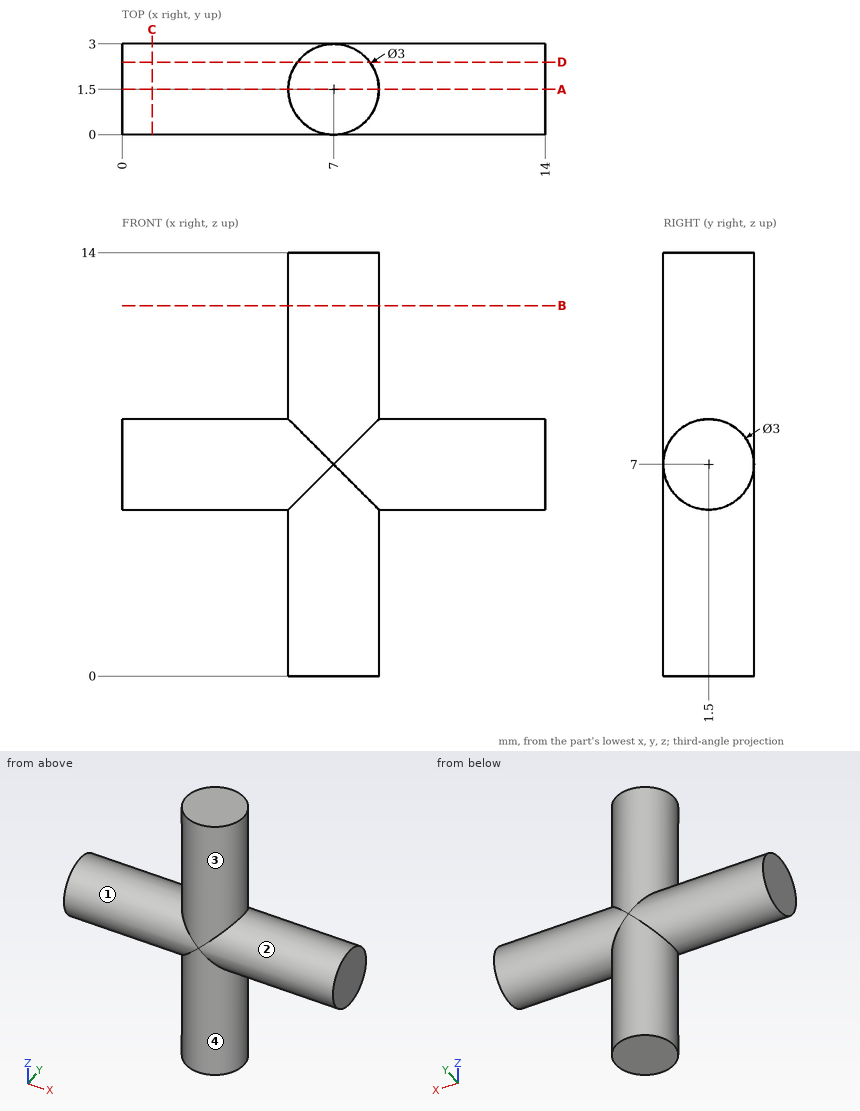
Check sheet for the drawn part. Datum: minimum x, y, z corner. Units: mm. A direction names the side the tool comes from. Coordinates: 2 decimals unless noted, no trailing zeros. Loops run counter-clockwise (first coordinate to the right, second up) from the corner with the lowest first, then second, coordinate; pieces in that order, holes last. Notation, with made-up numbers: (5, -8.5) - (62, -8.5) arc R14 ccw to (62, 9.5) - close; hole circle Ø3 at (-30, 55). An arc over 180 degrees is marked (long way). Put each result on its own line as item: value.
Item 1: Gauge pin test, flat end, axial feed: pin 1 Ø1 at (x, z) = (4, 1.5) entering from +Y. Record the tip position at first contact, or that the pin passes through.
Conclusion:
pin 1: passes through
Item 2: Set-up check for the marked faces 1, 2, 3 and 4: record each of +Z, -Z, +X, -X, +Y, -Y from which the full face is reachable in a straight line by a thin tool's end or side.
Conclusion:
face 1: -X
face 2: +X
face 3: +Z
face 4: -Z
Item 3: Section check C-C (x = 1). Enter the section's corners in (y, z), then the cut area to 3 significant figures.
Conclusion:
outline: circle Ø3 at (1.5, 7)
area: 7.07 mm2
Item 4: Section check A-A (y = 1.5). Enter the section's corners in (x, z).
Conclusion:
outline: (0, 5.5) - (5.5, 5.5) - (5.5, 0) - (8.5, 0) - (8.5, 5.5) - (14, 5.5) - (14, 8.5) - (8.5, 8.5) - (8.5, 14) - (5.5, 14) - (5.5, 8.5) - (0, 8.5) - close
Item 5: Section check D-D (y = 2.4). Enter the section's corners in (x, z).
Conclusion:
outline: (0, 5.8) - (5.8, 5.8) - (5.8, 0) - (8.2, 0) - (8.2, 5.8) - (14, 5.8) - (14, 8.2) - (8.2, 8.2) - (8.2, 14) - (5.8, 14) - (5.8, 8.2) - (0, 8.2) - close
Item 6: Scan lines: line 1 along Z through (x, y) = (11.5, 1.6); line 2 along X through (y, z) = (1.1, 9.75); line 3 along Z through (x, y) = (2.25, 0.25). Record each from-to range of solid material in increasing order.
Conclusion:
line 1: z = 5.5 to 8.5
line 2: x = 5.55 to 8.45
line 3: z = 6.17 to 7.83
Item 7: Section check B-B (z = 12.25). Enter the section's corners in (x, y).
Conclusion:
outline: circle Ø3 at (7, 1.5)
